Input: part model. Units: mm. Frame: model coordinates. Round coordinates to 2 decimals unless told otherwise and drop trailing zeros. Loops run counter-clockwise (first coordinate to the right, second up) from the corner with the lowest first, then second, coordinate; pieces in that order, holes last. Notation, with made-up numbers: (65.25, 57.25) - (114.25, 57.25) arc R28 cw to (114.25, 87.25) - close; hole circle Ø7 at (44.5, 6). An arc over 180 degrees is marked (long way). Use CSV: the item, a comma, the result in double quotes. Start each with the question number.
1. Cut plane A-A (z = 60.5). Return loops of the section in (x, y), and give its area (3 significant figures).
2. Pull-direction query (Z, two-part tool) for faces 1 (the cylindrical face through (-475.785, 3.057, 74.02)), 2 (the flat face through (6, 6.2, 20)), 3 (the cylindrical face through (-501.878, 3.143, -59.236)), 4 (the cylindrical face through (-10.316, 3.143, 7.91)); classes: +Z half, -Z half, draft (parallel to the pull), parting line (faces both ways), or undercut.
3. Cut plane B-B (x = -270). Return loops of the section in (y, z), and give its area (3 significant figures).
4. Material intervals for probe 1 along Z at (x, y) = (-67.5, 2.75); probe 2 along Z at (x, y) = (0, 2.75); probe 3 along X at (y, z) = (2.5, 48), sorted ascending. Write a range as from..to.
5. Pin query (flat end, axial travel): P1, Ø3, axis at x = 41.5, y = 3.5, coming from the -Z side; P2, Ø3, axis at y = 4, z = -28.5, coming from the +X side; P3, Ø3, axis at y = 1.5, z = -61.5, coming from the -X side. Return the tip coordinate at first contact, or that it passes through.
Autodesk Inventor part; units mm, degrees
ref_plane "YZ Plane" through (0, 0, 0) normal (1, 0, 0) x (0, 1, 0)
ref_plane "XZ Plane" through (0, 0, 0) normal (0, 1, 0) x (-1, 0, 0)
ref_plane "XY Plane" through (0, 0, 0) normal (0, 0, 1) x (1, 0, 0)
sketch "Sketch1" plane through (0, 0, 0) normal (0, 1, 0) x (-1, 0, 0)
  line L0 (432, 86) -> (-432, 86)
  line L1 (-432, -86) -> (432, -86)
  arc A0 (432, -86) -> (432, 86) centre (432, 0) ccw
  arc A1 (-432, 86) -> (-432, -86) centre (-432, 0) ccw
  point P0 (0, 0)
  dimension "d4" = 432
  dimension "d5" = 864
  dimension "d7" = 86
  dimension "d107" = 172
extrude "Extrusion1" add sketch "Sketch1" along normal blind 6.2
sketch "Sketch4" plane through (0, 6.2, 0) normal (0, 1, 0) x (1, 0, 0)
  line L0 (-659.0781, -10) -> (-659.0781, 10)
  line L1 (670.9769, 10) -> (670.9769, -10)
  line L2 (-10, 220.6364) -> (10, 220.6364)
  line L3 (-125, -216.3636) -> (-145, -216.3636)
  line L4 (-145, 220.6364) -> (-125, 220.6364)
  line L5 (-260, -216.3636) -> (-280, -216.3636)
  line L6 (-280, 220.6364) -> (-260, 220.6364)
  line L7 (145, -216.3636) -> (125, -216.3636)
  line L8 (125, 220.6364) -> (145, 220.6364)
  line L9 (280, -216.3636) -> (260, -216.3636)
  line L10 (260, 220.6364) -> (280, 220.6364)
  line L11 (395, 220.6364) -> (415, 220.6364)
  line L12 (-432, -86) -> (432, -86)
  line L13 (432, 86) -> (-432, 86)
  line L14 (395, 86) -> (395, 220.6364)
  line L15 (415, 220.6364) -> (415, 86)
  line L16 (280, -86) -> (280, -216.3636)
  line L17 (260, -216.3636) -> (260, -86)
  line L18 (280, 220.6364) -> (280, 86)
  line L19 (260, 86) -> (260, 220.6364)
  line L20 (145, -86) -> (145, -216.3636)
  line L21 (125, -216.3636) -> (125, -86)
  line L22 (145, 220.6364) -> (145, 86)
  line L23 (125, 86) -> (125, 220.6364)
  line L24 (10, 220.6364) -> (10, 86)
  line L25 (-10, 86) -> (-10, 220.6364)
  line L26 (-125, -86) -> (-125, -216.3636)
  line L27 (-145, -216.3636) -> (-145, -86)
  line L28 (-125, 220.6364) -> (-125, 86)
  line L29 (-145, 86) -> (-145, 220.6364)
  line L30 (-260, -86) -> (-260, -216.3636)
  line L31 (-280, -216.3636) -> (-280, -86)
  line L32 (-260, 220.6364) -> (-260, 86)
  line L33 (-280, 86) -> (-280, 220.6364)
  arc A0 (395, 86) -> (415, 86) centre (405, 86) ccw
  arc A1 (260, 86) -> (280, 86) centre (270, 86) ccw
  arc A2 (125, 86) -> (145, 86) centre (135, 86) ccw
  arc A3 (-10, 86) -> (10, 86) centre (0, 86) ccw
  arc A4 (-145, 86) -> (-125, 86) centre (-135, 86) ccw
  arc A5 (-280, 86) -> (-260, 86) centre (-270, 86) ccw
  arc A6 (-260, -86) -> (-280, -86) centre (-270, -86) ccw
  arc A7 (-125, -86) -> (-145, -86) centre (-135, -86) ccw
  arc A8 (145, -86) -> (125, -86) centre (135, -86) ccw
  arc A9 (280, -86) -> (260, -86) centre (270, -86) ccw
  arc A10 (518, 10) -> (518, -10) centre (518, 0) ccw
  arc A11 (-518, -10) -> (-518, 10) centre (-518, 0) ccw
  line L34 (-659.0781, 10) -> (-518, 10)
  line L35 (517.4166, 10) -> (670.9769, 10)
  line L36 (670.9769, -10) -> (518, -10)
  line L37 (-518, -10) -> (-659.0781, -10)
  circle A12 centre (-480, 48) radius 4
  circle A13 centre (-337.5, 76) radius 4
  circle A14 centre (337.5, 76) radius 4
  circle A15 centre (480, 48) radius 4
  circle A16 centre (480, -48) radius 4
  circle A17 centre (337.5, -76) radius 4
  circle A18 centre (-337.5, -76) radius 4
  circle A19 centre (-480, -48) radius 4
  arc A20 (-432, 86) -> (-432, -86) centre (-432, 0) ccw
  line L38 (10, -86) -> (10, -216.3636)
  line L39 (-10, -216.3636) -> (-10, -86)
  arc A21 (10, -86) -> (-10, -86) centre (0, -86) ccw
  line L40 (-10, -216.3636) -> (10, -216.3636)
  line L41 (-415, 220.6364) -> (-395, 220.6364)
  line L42 (-395, 220.6364) -> (-395, 86)
  line L43 (-415, 86) -> (-415, 220.6364)
  arc A22 (-415, 86) -> (-395, 86) centre (-405, 86) ccw
  line L44 (415, -216.3636) -> (395, -216.3636)
  line L45 (415, -86) -> (415, -216.3636)
  line L46 (395, -216.3636) -> (395, -86)
  arc A23 (415, -86) -> (395, -86) centre (405, -86) ccw
  line L47 (-395, -216.3636) -> (-415, -216.3636)
  line L48 (-395, -86) -> (-395, -216.3636)
  line L49 (-415, -216.3636) -> (-415, -86)
  arc A24 (-395, -86) -> (-415, -86) centre (-405, -86) ccw
  line L50 (-432, 0) -> (-518, 0)
  circle A25 centre (-67.5, 76) radius 4
  circle A26 centre (67.5, 76) radius 4
  circle A27 centre (67.5, -76) radius 4
  circle A28 centre (-67.5, -76) radius 4
  point P0 (480, -91)
  point P1 (480, 91)
  point P2 (-395, 86)
  point P3 (-395, 86)
  dimension "d18" = 20
  dimension "d54" = 76
  dimension "d55" = 48
  dimension "d59" = 48
  dimension "d60" = 76
  dimension "d73" = 8
  dimension "d109" = 135
  dimension "d110" = 135
  dimension "d111" = 135
  dimension "d112" = 135
  dimension "d113" = 135
  dimension "d115" = 135
  dimension "d116" = 20
  dimension "d120" = 48
  dimension "d121" = 38
  dimension "d122" = 38
  dimension "d123" = 48
  dimension "d124" = 38
  dimension "d125" = 38
  dimension "d130" = 76
  dimension "d131" = 76
  dimension "d144" = 76
  dimension "d145" = 76
  dimension "d146" = 76
  dimension "d147" = 76
  dimension "d149" = 57.5
  dimension "d150" = 57.5
  dimension "d151" = 57.5
  dimension "d152" = 57.5
  dimension "d153" = 57.5
  dimension "d154" = 57.5
  dimension "d155" = 57.5
  dimension "d156" = 57.5
extrude "Extrusion3" cut sketch "Sketch4" against normal through all
sketch "Sketch10" plane through (0, 6.2, 0) normal (0, 1, 0) x (1, 0, 0)
  circle A0 centre (0, 0) radius 13
extrude "Extrusion7" cut sketch "Sketch10" against normal through all
sketch "Sketch13" plane through (0, 6.2, 0) normal (0, 1, 0) x (1, 0, 0)
  line L0 (-460, 0) -> (-451, 0)
  arc A0 (-432, 86) -> (-517.4186, 9.9831) centre (-432, 0) ccw
  arc A1 (-436.8451, 85.8634) -> (-451, 70.8872) centre (-436, 70.8872) ccw
  line L1 (-460, 76.909) -> (-460, 0)
  line L2 (-451, 0) -> (-451, 70.8872)
  arc A2 (-451, 90.6568) -> (-460, 76.909) centre (-445, 76.909) ccw
  arc A3 (-517.4186, -9.9831) -> (-432, -86) centre (-432, 0) ccw
  line L3 (-436.8451, 85.8634) -> (-436.8451, 93.1)
  line L4 (-451, 90.6568) -> (-436.8451, 93.1)
  point P0 (0, 0)
  dimension "d163" = 9
  dimension "d167" = 30
  dimension "d168" = 460
  dimension "d169" = 15
  dimension "d175" = 0
extrude "Extrusion10" cut sketch "Sketch13" against normal through all
sketch "Sketch14" plane through (0, 6.2, 0) normal (0, 1, 0) x (1, 0, 0)
  line L0 (-451, 0) -> (-460, 0)
  line L1 (-460, 0) -> (-515.1777, -9.5935) construction
  line L2 (-460, 0) -> (-460, 76.909)
  line L3 (-460, 0) -> (-486.8762, 73.8417)
  arc A0 (-459.2589, 81.5656) -> (-517.4186, 9.9831) centre (-432, 0) ccw
  arc A1 (-517.4186, -9.9831) -> (-432, -86) centre (-432, 0) ccw
  line L4 (-280, 86) -> (-395, 86)
  line L5 (-395, -86) -> (-280, -86)
  line L6 (-460, 0) -> (-507.9899, -40.2683)
  line L7 (-460, 0) -> (-536.3277, 0) construction
  line L8 (-459.2589, 81.5656) -> (-459.2589, 87.869)
  arc A2 (-460, 87.6356) -> (-486.8762, 73.8417) centre (-434.6538, 5.1707) ccw
  line L9 (-517.4186, -9.9831) -> (-519.5785, -9.9831)
  line L10 (-517.4186, 9.9831) -> (-520.7839, 9.9831)
  arc A3 (-519.6047, -9.8704) -> (-519.5983, -9.8714) centre (-518, 0) ccw
  arc A4 (-459.2589, 87.869) -> (-520.7839, 9.9831) centre (-434.6234, 5.1651) ccw
  arc A5 (-519.5983, -9.8714) -> (-507.9899, -40.2683) centre (-434.6234, 5.1651) ccw
  arc A6 (-517.4186, -9.9831) -> (-507.9899, -40.2683) centre (-432, 0) ccw
  arc A7 (-459.2589, 81.5656) -> (-517.4186, 9.9831) centre (-432, 0) ccw
  point P0 (0, 0)
  point P1 (-484.7279, 67.9394)
  dimension "d182" = 40
  dimension "d183" = 70
extrude "Extrusion11" add sketch "Sketch14" against normal up to surface (6.2 mm away)
properties part number "1312_Former Middle_V1" material "Aluminum 6061"
Established:
1,outline,"(-493.12, 0) - (493.12, 0) - (493.12, 6.2) - (-493.12, 6.2) - close"
1,area,"6,110 mm2"
2,face 1,"+Z half"
2,face 2,"draft"
2,face 3,"-Z half"
2,face 4,"undercut"
3,outline,"(0, -76) - (6.2, -76) - (6.2, 76) - (0, 76) - close"
3,area,"942 mm2"
4,probe 1,"z = -86..-80, -72..72, 80..86"
4,probe 2,"z = -76..-13, 13..76"
4,probe 3,"x = -503.36..-484, -476..476, 484..503.36"
5,P1,"stops at z = -86"
5,P2,"stops at x = 513.65"
5,P3,"stops at x = -501.26"
